```python
from build123d import *

# Parameters (mm, degrees)
F0_W     = 114.3
F0_H     = 50.8
F0_R     = 15.24
F1_DEPTH = 25.4
F4_DEPTH = 50.801
F5_R     = 7.62
F6_DEPTH = 25.4


# Not quite as in the source:
# - ends of sketch curves that miss each other by under 0.0002 mm in the source are joined


with BuildPart() as f1:
    # F0 (on Top) → F1 (new body)
    with BuildSketch(Plane.XY):
        Rectangle(F0_W, F0_H)
        Circle(F0_R, mode=Mode.SUBTRACT)
    extrude(amount=F1_DEPTH)

    # F3 (on face) → F4 (cut, through all)
    with BuildSketch(Plane(origin=(0, 25.4, 0), x_dir=(-1, 0, 0), z_dir=(0, 1, 0))):
        Polygon((27.7357548475, 0), (42.9095774889, 0), (47.6239210906, 8.1654826425), (23.0214107298, 8.1654835362), align=None)
    extrude(amount=-F4_DEPTH, mode=Mode.SUBTRACT)

    # F5 (on face) → F6 (join)
    with BuildSketch(Plane.YZ.offset(57.15)):
        with Locations((0, 12.7)):
            Circle(F5_R)
    extrude(amount=F6_DEPTH)


solid = f1.part
```
The listing builds one solid part. Answer for the finished solid, in the listing's coordinates (mm). A direction names the side the tool comes from. Give positions to 0.01 mm unless a question says otherwise; leave off trailing zeros. Loops run counter-clockwise (first coordinate to the right, second up) from the corner with the lowest first, then second, coordinate; pieces in that order, holes last. Notation, with made-up numbers: M -22.5,13 L 25.5,13 A18 ccw 25.5,33 Z; hole C -5.75,-2.75 d6. An arc over 180 degrees is marked long. One line per item, written item: value.
1. Find the intervals of material crossed by probe 1 along Y at (x, z) = (0, 13.25); probe 2 along X at (y, z) = (-7.5, 3.75); probe 3 along X at (y, z) = (-6, 7.5), in increasing order.
Found:
probe 1: -25.4 to -15.24, 15.24 to 25.4
probe 2: -57.15 to -45.07, -25.57 to -13.27, 13.27 to 57.15
probe 3: -57.15 to -47.24, -23.41 to -14.01, 14.01 to 57.15
2. For faces 5 (the face through (-45.234, 0.356, 4.026)), 6 (the face through (-1, 17, 25.4)), determine the directions among +Z, -Z, +X, -X, +Y, -Y from which every point of the face is accessible in a straight line to the end or side of a thin tool.
Found:
face 5: +Y, -Y
face 6: +Z, +X, -X, +Y, -Y
3. Each of these flat-tipped pins is pushed along its axis until it touches: P1, Ø6, axis at y = 17.5, z = 11.5, coming from the +X side; P2, Ø7.5, axis at x = -34.5, y = 0, coming from the -Z side. Where does it stop, or does it pass through?
Found:
P1: x = 57.15
P2: z = 8.17
4. Section C-C on x = 0 is taken. Determine the outline of the cut face in (y, z).
Found:
outline: M -25.4,0 L -15.24,0 L -15.24,25.4 L -25.4,25.4 Z; M 15.24,0 L 25.4,0 L 25.4,25.4 L 15.24,25.4 Z
5. For a pull along X with two mould halves and no side action, classify faces 1 (the face through (-25.346, 0.356, 4.14)), 2 (the face through (69.672, -0.992, 20.255)), 3 (the face through (-35, 0, 8.165)), 4 (the face through (57.15, -6, 7)) as pulls with the +X half, pulls with the -X half, needs draft (parallel to the pull), parting line crosses it, or undercut.
Found:
face 1: undercut
face 2: needs draft
face 3: undercut
face 4: pulls with the +X half
6. Section B-B on z = 23.25 is taken. Determine the outline of the cut face in (x, y), plus the area to 3 significant figures.
Found:
outline: M -57.15,-25.4 L 57.15,-25.4 L 57.15,25.4 L -57.15,25.4 Z; hole C 0,0 d30.48
area: 5,080 mm^2
7. Section A-A on y = 0 is taken. Determine the outline of the cut face in (x, z).
Found:
outline: M -57.15,0 L -42.91,0 L -47.62,8.17 L -23.02,8.17 L -27.74,0 L -15.24,0 L -15.24,25.4 L -57.15,25.4 Z; M 15.24,0 L 57.15,0 L 57.15,5.08 L 82.55,5.08 L 82.55,20.32 L 57.15,20.32 L 57.15,25.4 L 15.24,25.4 Z
8. Section D-D on y = -20 is taken. Determine the outline of the cut face in (x, z), plus the area to 3 significant figures.
Found:
outline: M -57.15,0 L -42.91,0 L -47.62,8.17 L -23.02,8.17 L -27.74,0 L 57.15,0 L 57.15,25.4 L -57.15,25.4 Z
area: 2,740 mm^2
